from build123d import *

# Parameters (mm, degrees)
F1_DEPTH  = 2
F2_W      = 2
F2_H      = 33
F2_H_2    = 38
F3_DEPTH  = 75
F5_DEPTH  = 2
F6_W      = 2.5
F6_H      = 87.5
F7_DEPTH  = 7.5
F9_DEPTH  = 102.501
F11_DEPTH = 84.001
F13_DEPTH = 98
F15_DEPTH = 2.5
F17_DEPTH = 2.5
F19_DEPTH = 2.5
F21_DEPTH = 2.5
F23_W     = 30.666666667
F23_H     = 0.8284271247
F23_W_2   = 30.6666666667
F23_H_2   = 35.5
F24_DEPTH = 2


# Not quite as in the source:
# - a feature names something its author has since deleted; it is built from what else it names


with BuildPart() as f1:
    # F0 (on Right) → F1 (new body)
    with BuildSketch(Plane.YZ):
        Polygon((0, 10), (10, 0), (100, 0), (100, 37.5), (100, 45), (15, 45), (0, 30), align=None)
        Polygon((100, 45), (100, 37.5), (102.5, 40), (102.5, 45), align=None)
    extrude(amount=-F1_DEPTH)

    # F2 (on face) → F3 (join)
    with BuildSketch(Plane.YZ):
        Polygon((2, 30), (0, 30), (0, 10), (10, 0), (100, 0), (100, 37.5), (102.5, 40), (102.5, 45), (100.5, 45), (100.5, 40.8284271247), (98, 38.3284271247), (98, 2), (67.3333333333, 2), (65.3333333333, 2), (34.6666666667, 2), (32.6666666667, 2), (10.8284271247, 2), (2, 10.8284271247), align=None)
        with Locations((33.6666666667, 18.5)):
            Rectangle(F2_W, F2_H)
        with Locations((66.3333333333, 21)):
            Rectangle(F2_W, F2_H_2)
    extrude(amount=F3_DEPTH)

    # F4 (on face) → F5 (join)
    with BuildSketch(Plane.YZ.offset(75)):
        Polygon((100.5, 45), (15, 45), (0, 30), (0, 10), (10, 0), (100, 0), (100, 37.5), (102.5, 40), (102.5, 45), align=None)
    extrude(amount=F5_DEPTH)

    # F6 (on face) → F7 (join)
    with BuildSketch(Plane.XY.offset(45)):
        with Locations((-3.25, 58.75)):
            Rectangle(F6_W, F6_H)
        with Locations((78.25, 58.75)):
            Rectangle(F6_W, F6_H)
    extrude(amount=-F7_DEPTH)

    # F8 (on face) → F9 (cut, through all)
    with BuildSketch(Plane(origin=(0, 102.5, 0), x_dir=(-1, 0, 0), z_dir=(0, 1, 0))):
        Polygon((-79.5, 37.5), (-77, 37.5), (-79.5, 40), align=None)
        Polygon((4.5, 40), (2, 37.5), (4.5, 37.5), align=None)
    extrude(amount=-F9_DEPTH, mode=Mode.SUBTRACT)

    # F10 (on face) → F11 (cut, through all)
    with BuildSketch(Plane.YZ.offset(79.5)):
        Polygon((100, 37.5), (102.5, 37.5), (102.5, 40), align=None)
    extrude(amount=-F11_DEPTH, mode=Mode.SUBTRACT)

    # F12 (on face) → F13 (cut, through all)
    with BuildSketch(Plane.XZ):
        Polygon((77, 45), (75, 45), (0, 45), (-2, 45), (-2.5, 45), (-2.5, 40.8284271247), (0, 38.3284271247), (75, 38.3284271247), (75.3564065228, 38.6848336475), (77.5, 40.8284271247), (77.5, 45), align=None)
    extrude(amount=-F13_DEPTH, mode=Mode.SUBTRACT)

    # F14 (on face) → F15 (cut, through all)
    with BuildSketch(Plane(origin=(75, 0, 0), x_dir=(0, -1, 0), z_dir=(-1, 0, 0))):
        Polygon((-100.5, 40.8284271247), (-98, 38.3284271247), (-98, 45), (-100.5, 45), align=None)
    extrude(amount=-F15_DEPTH, mode=Mode.SUBTRACT)

    # F16 (on face) → F17 (join, through all)
    with BuildSketch(Plane(origin=(0, 98, 0), x_dir=(-1, 0, 0), z_dir=(0, 1, 0))):
        Polygon((-77.5, 38.3284271247), (-75, 38.3284271247), (-77.5, 40.8284271247), align=None)
    extrude(amount=F17_DEPTH)

    # F18 (on face) → F19 (cut, through all)
    with BuildSketch(Plane.YZ):
        Polygon((100.5, 40.8284271247), (100.5, 45), (98, 45), (98, 38.3284271247), align=None)
    extrude(amount=-F19_DEPTH, mode=Mode.SUBTRACT)

    # F20 (on face) → F21 (join, through all)
    with BuildSketch(Plane(origin=(0, 98, 0), x_dir=(-1, 0, 0), z_dir=(0, 1, 0))):
        Polygon((2.5, 38.3284271247), (2.5, 40.8284271247), (0, 38.3284271247), align=None)
    extrude(amount=F21_DEPTH)

    # F23 (on offset) → F24 (join)
    with BuildSketch(Plane.YZ.offset(36.5)):
        with Locations((82.6666666668, 37.9142135624)):
            Rectangle(F23_W, F23_H)
        with Locations((82.6666666667, 19.75)):
            Rectangle(F23_W_2, F23_H_2)
        Polygon((65.3333333333, 2), (65.3333333333, 37.5), (65.3333333333, 38.3284271247), (10, 38.3284271247), (10, 2.8284271247), (10.8284271247, 2), (32.6666666667, 2), (32.6666666667, 35), (34.6666666667, 35), (34.6666666667, 2), align=None)
        Polygon((10, 2.8284271247), (10, 38.3284271247), (2, 30), (2, 10.8284271247), align=None)
        Polygon((0, 30), (8.3284271248, 38.3284271248), (9.1642135624, 39.1642135624), (0, 48.3284271247), align=None)
        Polygon((2, 30), (10, 38.3284271247), (8.3284271251, 38.3284271247), (0, 30), align=None)
        Polygon((8.3284271251, 38.3284271247), (10, 38.3284271247), (9.1642135624, 39.1642135624), align=None)
    extrude(amount=F24_DEPTH)


solid = f1.part
Check sheet for the modelled part. Datum: model origin and axes. Units: mm. A direction names the side the tool comes from. Round coordinates to 2 decimals unless told otherwise and drop trailing zeros. Order: outer loops, then holes, each group sorted by start corner. A loop starts at its lowest first (then second) coordinate and runs counter-clockwise, first axis right, second up.
(1) Cross-section at A-A, the plane z = 19. Enter the section's corners in (x, y).
(2) Cross-section at D-D, the plane z = 42.5. Enter the section's corners in (x, y).
(3) Go/stop test with flat-tipped pins: P1, Ø1, axis at x = 15.5, y = 91.5, coming from the +Z side; P2, Ø6, axis at y = 15.5, z = 22, coming from the -X side; P3, Ø3.5, axis at x = 20, z = 43.5, coming from the -Y side. Record where each tip stops, or that it passes through.
(4) Cross-section at B-B, the plane x = 51.5. Enter the section's corners in (y, z).
(5) Cross-section at C-C, the plane y = 92. Enter the section's corners in (x, z).
(6) Draft check along Y on faces 3 (the flat face through (77, 49, 20)), 4 (the flat face through (18, 83, 2)), 5 (the flat face through (76, 5, 35)). Enter one of: pulls with the +Y half, pulls with the -Y half, needs draft (parallel to the pull), parting line crosses it, or undercut.
(7) Scan lines: probe 1 along Y at (x, z) = (15, 28); probe 2 along X at (y, z) = (96, 37); probe 3 along Y at (x, z) = (44, 31.5). Record each from-to range of solid material in increasing order.
(8) Access from +Z, -Z, +X, -X, +Y, -Y to the whole of each face (thin tool, end or side, straight path). Record for faces 1 (the flat face through (36.5, 32, 20)), 2 (the flat face through (79.5, 58, 43)).
Check sheet entries:
1. outline: (-2, 0) - (77, 0) - (77, 100) - (-2, 100) - close; hole (0, 2) - (36.5, 2) - (36.5, 32.67) - (0, 32.67) - close; hole (0, 34.67) - (36.5, 34.67) - (36.5, 65.33) - (0, 65.33) - close; hole (0, 67.33) - (36.5, 67.33) - (36.5, 98) - (0, 98) - close; hole (38.5, 2) - (75, 2) - (75, 32.67) - (38.5, 32.67) - close; hole (38.5, 34.67) - (75, 34.67) - (75, 65.33) - (38.5, 65.33) - close; hole (38.5, 67.33) - (75, 67.33) - (75, 98) - (38.5, 98) - close
2. outline: (-4.5, 15) - (-2.5, 15) - (-2.5, 100.5) - (77.5, 100.5) - (77.5, 15) - (79.5, 15) - (79.5, 102.5) - (-4.5, 102.5) - close; (36.5, 0) - (38.5, 0) - (38.5, 5.83) - (36.5, 5.83) - close
3. P1: stops at z = 2
3. P2: stops at x = -2
3. P3: stops at y = 100.5
4. outline: (0, 10) - (10, 0) - (100, 0) - (100, 37.5) - (102.5, 40) - (102.5, 45) - (100.5, 45) - (100.5, 40.83) - (98, 38.33) - (98, 2) - (67.33, 2) - (67.33, 38.33) - (65.33, 38.33) - (65.33, 2) - (34.67, 2) - (34.67, 35) - (32.67, 35) - (32.67, 2) - (10.83, 2) - (2, 10.83) - (2, 30) - (0, 30) - close
5. outline: (-4.5, 40) - (-2, 37.5) - (-2, 0) - (77, 0) - (77, 37.5) - (79.5, 40) - (79.5, 45) - (77.5, 45) - (77.5, 40.83) - (75, 38.33) - (75, 2) - (38.5, 2) - (38.5, 38.33) - (36.5, 38.33) - (36.5, 2) - (0, 2) - (0, 38.33) - (-2.5, 40.83) - (-2.5, 45) - (-4.5, 45) - close
6. face 3: needs draft
6. face 4: undercut
6. face 5: pulls with the -Y half
7. probe 1: y = 0 to 2, 32.67 to 34.67, 65.33 to 67.33, 98 to 100
7. probe 2: x = -2 to 0, 36.5 to 38.5, 75 to 77
7. probe 3: y = 32.67 to 34.67, 65.33 to 67.33, 98 to 100
8. face 1: +Z
8. face 2: +Z, -Z, +X, +Y, -Y
